Part model, mm, in its own coordinate system. Round coordinates to 2 decimals unless told otherwise and drop trailing zeros. Loops run counter-clockwise (first coordinate to the right, second up) from the corner with the lowest first, then second, coordinate; pieces in that order, holes last. Notation, with made-up numbers: M 10,38.5 L 34,38.5 A25 cw 34,71.5 Z; hole C 78.5,35.25 d11. An arc over 180 degrees is marked long. Answer as CSV lines item,"result". Start each with the question number.
Item 1: Band-saw the part on D-D (z = -0.7). Give the cut face in (x, y), and give its area (3 significant figures).
Item 2: Wall check: line 1 (X direction, y = -2, z = -1); line 2 (Y direction, x = -4.75, z = -0.85) (3 decimals); line 3 (Y direction, x = -2.75, z = -3.65). Give the ranges that are in metal, low to high.
Item 3: Band-saw the part on B-B (z = -1.4). Give the cut face in (x, y).
Item 4: Band-saw the part on C-C (x = -2.25). Give the cut face in (y, z).
Item 5: Drop flat-ended pins along their axis: pin 1 Ø2 at (x, y) = (-7, 3.5) entering from -Z; pin 2 Ø2 at (x, z) = (-1.5, -3) entering from -Y; pin 3 Ø1 at (x, y) = (-8, 3.5) entering from -Z. Give the stop position or say it passes through.
Item 6: Band-saw the part on A-A (y = 0). Give the cut face in (x, z).
```python
from build123d import *

# Parameters (mm, degrees)
F1_DEPTH = 12.5
F3_DEPTH = 4
F4_ANGLE = 90


with BuildPart() as f1:
    # F0 (on Top) → F1 (new body)
    with BuildSketch(Plane.XY):
        with BuildLine():
            Line((2, -4.95), (2, 4.95))
            ThreePointArc((2, 4.95), (-0.5303161858, 4.0842789494), (-2, 1.85))
            Line((-2, 1.85), (-2, -1.85))
            ThreePointArc((-2, -1.85), (-0.5303161858, -4.0842789494), (2, -4.95))
        make_face()
    extrude(amount=F1_DEPTH)

    # F2 (on face) → F3 (cut)
    with BuildSketch(Plane.YZ.offset(2)):
        with BuildLine():
            Line((0, 6.25), (-1.4279861962, 4.4469871261))
            ThreePointArc((-1.4279861962, 4.4469871261), (0, 3.95), (1.4279861962, 4.4469871261))
            Line((1.4279861962, 4.4469871261), (0, 6.25))
        make_face()
        with BuildLine():
            Line((1.4279861962, 8.0530128739), (0, 6.25))
            Line((0, 6.25), (1.4279861962, 4.4469871261))
            ThreePointArc((1.4279861962, 4.4469871261), (2.0705516476, 5.2485930525), (2.3, 6.25))
            ThreePointArc((2.3, 6.25), (2.0705516476, 7.2514069475), (1.4279861962, 8.0530128739))
        make_face()
        with BuildLine():
            Line((-1.4279861962, 8.0530128739), (0, 6.25))
            Line((0, 6.25), (1.4279861962, 8.0530128739))
            ThreePointArc((1.4279861962, 8.0530128739), (0, 8.55), (-1.4279861962, 8.0530128739))
        make_face()
        with BuildLine():
            ThreePointArc((-1.4279861962, 8.0530128739), (-2.3, 6.25), (-1.4279861962, 4.4469871261))
            Line((-1.4279861962, 4.4469871261), (0, 6.25))
            Line((0, 6.25), (-1.4279861962, 8.0530128739))
        make_face()
    extrude(amount=-F3_DEPTH, mode=Mode.SUBTRACT)


with BuildPart() as f1_1:
    # F4: moved
    add(f1.part.rotate(Axis((2, 0, 0), (0, -1, 0)), F4_ANGLE))


solid = f1_1.part
```
Answer block:
1,outline,"M -10.5,-4.89 L 2,-4.89 L 2,4.89 L -10.5,4.89 Z; hole C -4.25,0 d4.6"
1,area,"106 mm^2"
2,line 1,"x = -10.5 to -5.39, -3.11 to 2"
2,line 2,"y = -4.862 to -2.245, 2.245 to 4.862"
2,line 3,"y = -2.75 to -1.74, 1.74 to 2.75"
3,outline,"M -10.5,-4.71 L 2,-4.71 L 2,4.71 L -10.5,4.71 Z; hole C -4.25,0 d4.6"
4,outline,"M -4.95,0 A4.13 ccw -1.85,-4 L -1.14,-4 L -1.14,0 Z; M 1.14,-4 L 1.85,-4 A4.13 ccw 4.95,0 L 1.14,0 Z"
5,pin 1,"stops at z = -3.77"
5,pin 2,"stops at y = -4.43"
5,pin 3,"stops at z = -3.51"
6,outline,"M -10.5,-4 L -6.55,-4 L -6.55,0 L -10.5,0 Z; M -1.95,-4 L 2,-4 L 2,0 L -1.95,0 Z"
